Source: CAD feature listing. Evaluate the final solid. Frame: model axes, mm. Give positions to 0.01 mm unless a question says otherwise; leave off trailing zeros. Loops run counter-clockwise (first coordinate to the right, second up) from the corner with the lowest first, then second, coordinate; pieces in that order, holes last. Notation, with made-up numbers: M -39,87 L 1,87 A18 ccw 1,110 Z; hole C 24.25,-27.75 d7. An arc over 180 degrees is marked long. Put each result on its own line as item: value. Start each with the question number.
```python
from build123d import *

# Parameters (mm, degrees)
SKETCH_1_R                  = 1.5
SKETCH_1_W                  = 8
SKETCH_1_H                  = 6
EXTRUDE_1_DEPTH             = 3
HOLE_WIZARD_M3_1_AT_2_COUNT = 2
HOLE_WIZARD_M3_1_AT_2_PITCH = 14.76482306
HOLE_WIZARD_M3_1_AT_3_COUNT = 2
HOLE_WIZARD_M3_1_AT_3_PITCH = 26
FILLET_1_R                  = 1
CHAMFER_1_SIZE              = 5
FILLET_2_R                  = 3


with BuildPart() as part:
    # 草图1 → 凸台-拉伸1 (new body)
    with BuildSketch(Plane.XY):
        Polygon((36.5, -19), (-18, -19), (-18, 19), (21.5, 19), (21.5, 30), (36.5, 30), (36.5, 19), (36.5, 10), (30.5, 6.535898385), (30.5, -6.535898385), (36.5, -10), align=None)
        with Locations((-13, 16.5)):
            Circle(SKETCH_1_R, mode=Mode.SUBTRACT)
        with Locations((-13, -16.5)):
            Circle(SKETCH_1_R, mode=Mode.SUBTRACT)
        with Locations((13, -16.5)):
            Circle(SKETCH_1_R, mode=Mode.SUBTRACT)
        with Locations((13, 16.5)):
            Circle(SKETCH_1_R, mode=Mode.SUBTRACT)
        with Locations((32.5, -13)):
            Circle(SKETCH_1_R, mode=Mode.SUBTRACT)
        with Locations(Location((32.5, 13, 0), (0, 0, 180))):
            Circle(SKETCH_1_R, mode=Mode.SUBTRACT)
        with Locations((25.5, 0)):
            Circle(SKETCH_1_R, mode=Mode.SUBTRACT)
        with Locations((29, 26)):
            Circle(SKETCH_1_R, mode=Mode.SUBTRACT)
        with Locations((24.5, -11.5)):
            Rectangle(SKETCH_1_W, SKETCH_1_H, mode=Mode.SUBTRACT)
        with Locations((24.5, 11.5)):
            Rectangle(SKETCH_1_W, SKETCH_1_H, mode=Mode.SUBTRACT)
        Polygon((-13, -10.977083583), (-2.429475068, 0), (-13, 10.977083583), align=None, mode=Mode.SUBTRACT)
        Polygon((-10.570524932, -13.5), (0, -2.522916417), (10.570524932, -13.5), align=None, mode=Mode.SUBTRACT)
        Polygon((-10.570524932, 13.5), (0, 2.522916417), (10.570524932, 13.5), align=None, mode=Mode.SUBTRACT)
        Polygon((2.429475068, 0), (13, 10.977083583), (13, -10.977083583), align=None, mode=Mode.SUBTRACT)
    extrude(amount=EXTRUDE_1_DEPTH)

    # 草图2 → M3 六角凹锥坑螺钉的锥形沉头孔1 (revolve, cut)
    with BuildSketch(Plane(origin=(32.5, 13, 3), x_dir=(0, -1, 0), z_dir=(1, 0, 0))):
        Polygon((0, 0), (0, 3), (1.5, 3), (1.5, 1.86), (3.36, 0), align=None)
    hole_wizard_m3_1 = revolve(axis=Axis((32.5, 13, 9.35), (0, 0, -1)), mode=Mode.SUBTRACT)

    # M3 六角凹锥坑螺钉的锥形沉头孔1 at 2: M3 六角凹锥坑螺钉的锥形沉头孔1 ×2
    with Locations(*[Vector(-0.4740998230350173, -0.8804710999221754, 0) * (i * HOLE_WIZARD_M3_1_AT_2_PITCH) for i in range(1, HOLE_WIZARD_M3_1_AT_2_COUNT)]):
        add(hole_wizard_m3_1, mode=Mode.SUBTRACT)

    # M3 六角凹锥坑螺钉的锥形沉头孔1 at 3: M3 六角凹锥坑螺钉的锥形沉头孔1 ×2
    with Locations(*[(0, -i * HOLE_WIZARD_M3_1_AT_3_PITCH, 0) for i in range(1, HOLE_WIZARD_M3_1_AT_3_COUNT)]):
        add(hole_wizard_m3_1, mode=Mode.SUBTRACT)

    # 圆角1
    fillet_1_edges = [part.edges().sort_by_distance(p)[0] for p in [
        (-10.570524932, -13.5, 1.5),
        (10.570524932, -13.5, 1.5),
        (0, -2.522916417, 1.5),
        (13, -10.977083583, 1.5),
        (13, 10.977083583, 1.5),
        (2.429475068, 0, 1.5),
        (28.5, -8.5, 1.5),
        (20.5, -8.5, 1.5),
        (20.5, -14.5, 1.5),
        (28.5, -14.5, 1.5),
        (20.5, 14.5, 1.5),
        (20.5, 8.5, 1.5),
        (28.5, 8.5, 1.5),
        (28.5, 14.5, 1.5),
        (-13, 10.977083583, 1.5),
        (-13, -10.977083583, 1.5),
        (-2.429475068, 0, 1.5),
        (10.570524932, 13.5, 1.5),
        (-10.570524932, 13.5, 1.5),
        (0, 2.522916417, 1.5),
    ]]
    fillet(fillet_1_edges, radius=FILLET_1_R)

    # 倒角1
    chamfer_1_edges = [part.edges().sort_by_distance(p)[0] for p in [
        (21.5, 30, 1.5),
        (36.5, 30, 1.5),
    ]]
    chamfer(chamfer_1_edges, length=CHAMFER_1_SIZE)

    # 圆角2
    fillet_2_edges = [part.edges().sort_by_distance(p)[0] for p in [
        (36.5, 10, 1.5),
        (30.5, 6.535898385, 1.5),
        (30.5, -6.535898385, 1.5),
        (36.5, -10, 1.5),
    ]]
    fillet(fillet_2_edges, radius=FILLET_2_R)


solid = part.part
```
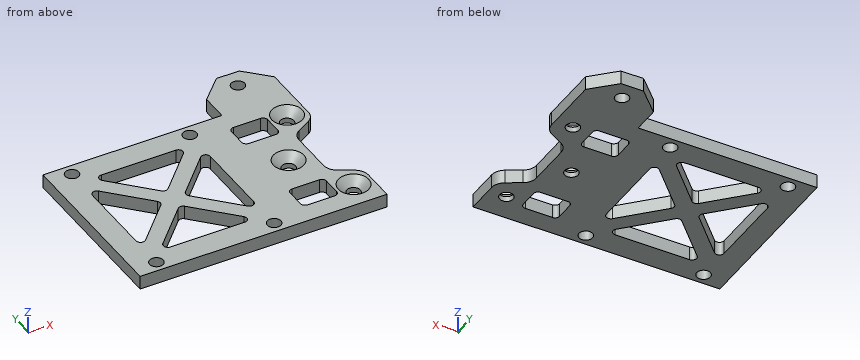
1. Section A-A, the plane x = 25.5. Output: boundary loops of the cut face in (y, z), plus the area to 3 significant figures.
2. Section C-C, the plane z = 0.45. State how many separate pieces and enclosed holes the cut face has, plus the area to 3 significant figures.
3. Section D-D, the plane x = 19. Output: boundary loops of the cut face in (y, z), plus the area to 3 significant figures.
4. Section B-B, the plane y = 0. Output: boundary loops of the cut face in (x, z).
5. Ray query, line 1 (X direction, y = 0, z = 0.7); line 2 (X direction, y = -10, z = 1); line 3 (Y direction, x = 32.5, z = 0.3). Return the intervals inside material, ascending.
6. Contact query for flat-ended pins moving along their axis: pin 1 (3.5 mm diameter, centred on x = 32.5, y = -13, fed in from +Z); pin 2 (2.5 mm diameter, centred on x = 32.5, y = 13, fed in from +Z); pin 3 (1.5 mm diameter, centred on x = 24, z = 2, fed in from +Y); pin 4 (1.5 mm diameter, centred on y = -2, z = 1.5, fed in from +X). Output: stop coordinate, or through.
Results found:
1. outline: M -19,0 L -14.5,0 L -14.5,3 L -19,3 Z; M -8.5,0 L -1.5,0 L -1.5,1.14 L -3.36,3 L -8.5,3 Z; M 1.5,0 L 8.5,0 L 8.5,3 L 3.36,3 L 1.5,1.14 Z; M 14.5,0 L 29,0 L 29,3 L 14.5,3 Z
1. area: 95.5 mm²
2. separate pieces: 1
2. enclosed holes: 14
2. area: 1,510 mm²
3. outline: M -19,0 L 19,0 L 19,3 L -19,3 Z
3. area: 114 mm²
4. outline: M -18,0 L -13,0 L -13,3 L -18,3 Z; M -2.82,0 L 2.82,0 L 2.82,3 L -2.82,3 Z; M 13,0 L 24,0 L 24,1.14 L 22.14,3 L 13,3 Z; M 27,0 L 30.5,0 L 30.5,3 L 28.86,3 L 27,1.14 Z
5. line 1: -18 to -13, -2.82 to 2.82, 13 to 24, 27 to 30.5
5. line 2: -18 to -7.2, 7.2 to 20.5, 28.5 to 35.95
5. line 3: -19 to -14.5, -11.5 to -7.69, 7.69 to 11.5, 14.5 to 29
6. pin 1: z = 1.39
6. pin 2: through
6. pin 3: y = 28.25
6. pin 4: x = 30.5
